```python
from build123d import *

# Parameters (mm, degrees)
SKETCH1_R           = 33.274
BOSS_EXTRUDE1_DEPTH = 57.15
CUT_EXTRUDE1_DEPTH  = 57.15
SKETCH4_R           = 120.65


with BuildPart() as part:
    # Sketch1 → Boss-Extrude1 (new body)
    with BuildSketch(Plane(origin=(0, 0, 0), x_dir=(1, 0, 0), z_dir=(0, 1, 0))):
        Circle(SKETCH1_R)
    extrude(amount=BOSS_EXTRUDE1_DEPTH)

    # Sketch2 → Cut-Extrude1 (cut)
    with BuildSketch(Plane.XZ):
        Polygon((-15.323636661, -1.510781079), (-6.353443536, -14.026049167), (8.970193125, -12.515268087), (15.323636661, 1.510781079), (6.353443536, 14.026049167), (-8.970193125, 12.515268087), align=None)
    extrude(amount=-CUT_EXTRUDE1_DEPTH, mode=Mode.SUBTRACT)

    # Sketch4 → Cut-Revolve2 (revolve, cut)
    with BuildSketch(Plane.XY):
        with Locations((-139.52982337, 57.15)):
            Circle(SKETCH4_R)
    revolve(axis=Axis((0, 0, 0), (0, 1, 0)), mode=Mode.SUBTRACT)


solid = part.part
```
Could you check a few things on this model? Use its own coordinates, in mm. A direction names the side the tool comes from. Coordinates: 2 decimals unless noted, no trailing zeros. Loops run counter-clockwise (first coordinate to the right, second up) from the corner with the lowest first, then second, coordinate; pieces in that order, holes last.
1) Imagine slicing it at A-A (y = 15). List the corners of the cut face in (x, z) for me.
Reported:
outline: circle Ø52.96 at (0, 0); hole (-15.32, -1.51) - (-6.35, -14.03) - (8.97, -12.52) - (15.32, 1.51) - (6.35, 14.03) - (-8.97, 12.52) - close
2) Will these pins go through, and if not, where does the flat tip stop? pin 1 Ø4 at (x, y) = (-7, 10) entering from -Z; pin 2 Ø4 at (y, z) = (24.5, -5.5) entering from +X; pin 3 Ø1.5 at (y, z) = (19, -23.5) entering from -X.
Reported:
pin 1: stops at z = -28.61
pin 2: stops at x = 23.46
pin 3: stops at x = -10.64
3) Thinking about a two-plate mould opening in X: for faces 1 (the face through (10, 57.15, 10)), 2 (the face through (12.102, 28.175, -5.6)), 3 (the face through (-1.2, 28.17, 13.28)), which applies, released by +X, released by -X, zero draft, split by the parting line, or undercut?
Reported:
face 1: zero draft
face 2: undercut
face 3: undercut
4) Which directions (+Z, -Z, +X, -X, +Y, -Y) give clear straight access to the entire face, cutting with the end or side of a thin tool? Please do faces 4 (the face through (1.2, 28.17, -13.28)), 5 (the face through (0, 0, 14)).
Reported:
face 4: +Y, -Y
face 5: +Z, -Z, +X, -X, -Y
5) Imagine slicing it at B-B (y = 23.5). List the corners of the cut face in (x, z) for me, and give its area (3 significant figures).
Reported:
outline: circle Ø47.33 at (0, 0); hole (-15.32, -1.51) - (-6.35, -14.03) - (8.97, -12.52) - (15.32, 1.51) - (6.35, 14.03) - (-8.97, 12.52) - close
area: 1,140 mm2
6) Please list where these lines run through material, in increasing order: line 1 along Z through (x, y) = (-2.5, 33); line 2 along X through (y, z) = (16.5, -2.5); line 3 along X through (y, z) = (25, -11).
Reported:
line 1: z = -21.17 to -13.65, 13.15 to 21.17
line 2: x = -25.81 to -14.61, 13.51 to 25.81
line 3: x = -20.47 to -8.52, 9.66 to 20.47
